CAD build for the part. Positions are in the model's coordinates, mm. A direction names the side the tool comes from. Coordinates: 2 decimals unless noted, no trailing zeros. Order: outer loops, then holes, each group sorted by start corner. A loop starts at its lowest first (then second) coordinate and runs counter-clockwise, first axis right, second up. Notation, with made-up numbers: (55, 14.5) - (114, 14.5) arc R17 cw to (114, 41.5) - close; hole circle Ø5 at (37, 29.5). An arc over 180 degrees is marked (long way). Write each question's results on one line, items separated by ' | '. Start each with the question number.
Q1. Band-saw the part on C-C, the plane z = 57. Write the cut outline in (x, y).
Q2. Band-saw the part on A-A, the plane z = 100. Write the cut outline in (x, y).
Q3. Pin check, flat tips, straight feed: P1, Ø2.5, axis at x = 14.5, z = 20, coming from the +Y side; P2, Ø20, axis at x = -4, z = 71.5, coming from the -Y side; P3, Ø3, axis at y = -41.5, z = 61.5, coming from the -X side; P4, Ø5.5, axis at x = -39.5, y = -55, coming from the -Z side. Stop position of each tip, or through.
Q4. Wall check: probe 1 along X at (y, z) = (-55, 87.9); probe 2 along Z at (x, y) = (14.5, -41.5); probe 3 along Z at (x, y) = (3, -48.75). Give the ranges that are in metal, low to high.
Q5. Band-saw the part on D-D, the plane y = -45.25. Write the cut outline in (x, z), then the cut area to 3 significant figures.
Q6. Band-saw the part on B-B, the plane x = -14.5. Write the cut outline in (y, z), then the cut area to 3 significant figures.
Q7. Which spindle directions (+Z, -Z, +X, -X, +Y, -Y) get a long thin tool onto all of the face, cutting with end or side? Do faces 1 (the flat face through (0, -50, 88)), 2 (the flat face through (0, -40, 83)), 3 (the flat face through (-20, -41, 47)), 4 (the flat face through (0, -49, 34.5)), 5 (the flat face through (0, -43, 19)). Say none if no direction does.
Q8. Pull direction Z, two halves, no side cores. Call faces 6 (the cylindrical face through (15.414, -39.958, 21.433)), 7 (the flat face through (0, -49, 28.5)), 8 (the flat face through (10, -54, 31)): released by +Z, released by -Z, zero draft, split by the parting line, or undercut.
```python
from build123d import *

# Parameters (mm, degrees)
BOX028_W          = 20
BOX028_H          = 20
BOX028_DEPTH      = 45
BOX029_W          = 20
BOX029_H          = 20
BOX029_DEPTH      = 45
BOX030_W          = 46
BOX030_H          = 20
BOX030_DEPTH      = 45
CYLINDER030_R     = 1.7
CYLINDER030_DEPTH = 50
CYLINDER031_R     = 1.7
CYLINDER031_DEPTH = 50
CYLINDER032_R     = 1.7
CYLINDER032_DEPTH = 50
CYLINDER033_R     = 1.7
CYLINDER033_DEPTH = 50
CYLINDER034_R     = 1.7
CYLINDER034_DEPTH = 50
CYLINDER035_R     = 1.7
CYLINDER035_DEPTH = 50
BOX026_W          = 90
BOX026_H          = 23
BOX026_DEPTH      = 6
BOX025_W          = 40
BOX025_H          = 6
BOX025_DEPTH      = 100
BOX027_W          = 40
BOX027_H          = 15
BOX027_DEPTH      = 6


with BuildPart() as cube025:
    # Box028 → Box028 (new body)
    with BuildSketch(Plane(origin=(-10, -51, 38), x_dir=(1, 0, 0), z_dir=(0, 0, 1))):
        with Locations((10, 10)):
            Rectangle(BOX028_W, BOX028_H)
    extrude(amount=BOX028_DEPTH)


with BuildPart() as cube026:
    # Box029 → Box029 (new body)
    with BuildSketch(Plane(origin=(-10, -68, 20), x_dir=(1, 0, 0), z_dir=(0, 0, 1))):
        with Locations((10, 10)):
            Rectangle(BOX029_W, BOX029_H)
    extrude(amount=BOX029_DEPTH)


with BuildPart() as cube027:
    # Box030 → Box030 (new body)
    with BuildSketch(Plane(origin=(-23, -68, 56), x_dir=(1, 0, 0), z_dir=(0, 0, 1))):
        with Locations((23, 10)):
            Rectangle(BOX030_W, BOX030_H)
    extrude(amount=BOX030_DEPTH)


with BuildPart() as mounting_hole:
    # Cylinder030 → Cylinder030 (new body)
    with BuildSketch(Plane(origin=(-14.5, 0, 20), x_dir=(1, 0, 0), z_dir=(0, -1, 0))):
        Circle(CYLINDER030_R)
    extrude(amount=CYLINDER030_DEPTH)


with BuildPart() as mounting_hole001:
    # Cylinder031 → Cylinder031 (new body)
    with BuildSketch(Plane(origin=(14.5, 0, 20), x_dir=(1, 0, 0), z_dir=(0, -1, 0))):
        Circle(CYLINDER031_R)
    extrude(amount=CYLINDER031_DEPTH)


with BuildPart() as mounting_hole002:
    # Cylinder032 → Cylinder032 (new body)
    with BuildSketch(Plane(origin=(-14.5, 0, 100), x_dir=(1, 0, 0), z_dir=(0, -1, 0))):
        Circle(CYLINDER032_R)
    extrude(amount=CYLINDER032_DEPTH)


with BuildPart() as mounting_hole003:
    # Cylinder033 → Cylinder033 (new body)
    with BuildSketch(Plane(origin=(14.5, 0, 100), x_dir=(1, 0, 0), z_dir=(0, -1, 0))):
        Circle(CYLINDER033_R)
    extrude(amount=CYLINDER033_DEPTH)


with BuildPart() as mounting_hole004:
    # Cylinder034 → Cylinder034 (new body)
    with BuildSketch(Plane(origin=(-39.5, -53, 58), x_dir=(1, 0, 0), z_dir=(0, 0, 1))):
        Circle(CYLINDER034_R)
    extrude(amount=CYLINDER034_DEPTH)


with BuildPart() as mounting_hole005:
    # Cylinder035 → Cylinder035 (new body)
    with BuildSketch(Plane(origin=(39.5, -53, 58), x_dir=(1, 0, 0), z_dir=(0, 0, 1))):
        Circle(CYLINDER035_R)
    extrude(amount=CYLINDER035_DEPTH)


with BuildPart() as cube023:
    # Box026 → Box026 (new body)
    with BuildSketch(Plane(origin=(-45, -58, 85.5), x_dir=(1, 0, 0), z_dir=(0, 0, 1))):
        with Locations((45, 11.5)):
            Rectangle(BOX026_W, BOX026_H)
    extrude(amount=BOX026_DEPTH)


with BuildPart() as fusion024:
    # Box025 → Box025 (new body)
    with BuildSketch(Plane(origin=(-20, -41, 10), x_dir=(1, 0, 0), z_dir=(0, 0, 1))):
        with Locations((20, 3)):
            Rectangle(BOX025_W, BOX025_H)
    extrude(amount=BOX025_DEPTH)

    # Fusion024: union Cube023
    add(cube023.part)


with BuildPart() as paste_extruder_psu_mounting_bracket:
    # Box027 → Box027 (new body)
    with BuildSketch(Plane(origin=(-20, -56, 28.5), x_dir=(1, 0, 0), z_dir=(0, 0, 1))):
        with Locations((20, 7.5)):
            Rectangle(BOX027_W, BOX027_H)
    extrude(amount=BOX027_DEPTH)

    # Fusion025: union Fusion024
    add(fusion024.part)

    # Cut035: cut mounting hole005
    add(mounting_hole005.part, mode=Mode.SUBTRACT)

    # Cut036: cut mounting hole004
    add(mounting_hole004.part, mode=Mode.SUBTRACT)

    # Cut037: cut mounting hole003
    add(mounting_hole003.part, mode=Mode.SUBTRACT)

    # Cut038: cut mounting hole002
    add(mounting_hole002.part, mode=Mode.SUBTRACT)

    # Cut039: cut mounting hole001
    add(mounting_hole001.part, mode=Mode.SUBTRACT)

    # Cut040: cut mounting hole
    add(mounting_hole.part, mode=Mode.SUBTRACT)

    # Cut041: cut Cube027
    add(cube027.part, mode=Mode.SUBTRACT)

    # Cut042: cut Cube026
    add(cube026.part, mode=Mode.SUBTRACT)

    # Cut043: cut Cube025
    add(cube025.part, mode=Mode.SUBTRACT)


with BuildPart() as paste_extruder_psu_mounting_bracket_1:
    # Cut043 placement: moved
    add(paste_extruder_psu_mounting_bracket.part.moved(Location((0, -2, 0))))


solid = paste_extruder_psu_mounting_bracket_1.part
```
Results below:
1) outline: (-20, -43) - (-10, -43) - (-10, -37) - (-20, -37) - close; (10, -43) - (20, -43) - (20, -37) - (10, -37) - close
2) outline: (-20, -43) - (-16.2, -43) - (-16.2, -37) - (-20, -37) - close; (-12.8, -43) - (12.8, -43) - (12.8, -37) - (-12.8, -37) - close; (16.2, -43) - (20, -43) - (20, -37) - (16.2, -37) - close
3) P1: passes through | P2: stops at y = -43 | P3: stops at x = -20 | P4: stops at z = 85.5
4) probe 1: x = -45 to -41.2, -37.8 to -23, 23 to 37.8, 41.2 to 45 | probe 2: z = 10 to 18.3, 21.7 to 98.3, 101.7 to 110 | probe 3: z = 28.5 to 34.5, 85.5 to 91.5
5) outline: (-45, 85.5) - (45, 85.5) - (45, 91.5) - (-45, 91.5) - close; (-20, 28.5) - (20, 28.5) - (20, 34.5) - (-20, 34.5) - close | area: 780 mm²
6) outline: (-58, 28.5) - (-43, 28.5) - (-43, 21.7) - (-37, 21.7) - (-37, 98.3) - (-43, 98.3) - (-43, 91.5) - (-50, 91.5) - (-50, 85.5) - (-43, 85.5) - (-43, 34.5) - (-58, 34.5) - close; (-43, 10) - (-37, 10) - (-37, 18.3) - (-43, 18.3) - close; (-43, 101.7) - (-37, 101.7) - (-37, 110) - (-43, 110) - close | area: 691 mm²
7) face 1: +Z, -Y | face 2: +Y, -Y | face 3: -Z, -X, +Y, -Y | face 4: +X, -X, -Y | face 5: -Z, +X, -X, -Y
8) face 6: undercut | face 7: released by -Z | face 8: zero draft
